```python
from build123d import *

# Parameters (mm, degrees)
BOSS_EXTRUDE1_DEPTH = 100
SKETCH4_W           = 90
SKETCH4_H           = 70
BOSS_EXTRUDE2_DEPTH = 45
SKETCH5_W           = 40
SKETCH5_H           = 45
CUT_EXTRUDE1_DEPTH  = 90
CUT_EXTRUDE2_DEPTH  = 70


with BuildPart() as part:
    # Sketch1 → Boss-Extrude1 (new body)
    with BuildSketch(Plane.XY):
        with BuildLine():
            Line((-52.117117117, 57.815315315), (-52.117117117, 2.815315315))
            Line((-52.117117117, 2.815315315), (47.882882883, 2.815315315))
            Line((47.882882883, 2.815315315), (47.882882883, -22.184684685))
            Line((47.882882883, -22.184684685), (-102.117117117, -22.184684685))
            Line((-102.117117117, -22.184684685), (-102.117117117, 2.815315315))
            Line((-102.117117117, 2.815315315), (-102.117117117, 57.815315315))
            ThreePointArc((-102.117117117, 57.815315315), (-77.117117117, 82.815315315), (-52.117117117, 57.815315315))
        make_face()
        with BuildLine():
            Line((-67.117117117, 57.815315315), (-67.117117117, 2.815315315))
            ThreePointArc((-67.117117117, 2.815315315), (-77.117117117, -7.184684685), (-87.117117117, 2.815315315))
            Line((-87.117117117, 2.815315315), (-87.117117117, 57.815315315))
            ThreePointArc((-87.117117117, 57.815315315), (-77.117117117, 67.815315315), (-67.117117117, 57.815315315))
        make_face(mode=Mode.SUBTRACT)
    extrude(amount=-BOSS_EXTRUDE1_DEPTH)

    # Sketch4 → Boss-Extrude2 (add)
    with BuildSketch(Plane(origin=(0, 2.815315315, 0), x_dir=(1, 0, 0), z_dir=(0, 1, 0))):
        with Locations((-7.117117117, 50)):
            Rectangle(SKETCH4_W, SKETCH4_H)
    extrude(amount=BOSS_EXTRUDE2_DEPTH)

    # Sketch5 → Cut-Extrude1 (cut)
    with BuildSketch(Plane(origin=(37.882882883, 0, 0), x_dir=(0, 0, -1), z_dir=(1, 0, 0))):
        with Locations((50, 25.315315315)):
            Rectangle(SKETCH5_W, SKETCH5_H)
    extrude(amount=-CUT_EXTRUDE1_DEPTH, mode=Mode.SUBTRACT)

    # Sketch6 → Cut-Extrude2 (cut)
    with BuildSketch(Plane.XY.offset(-15)):
        Polygon((-52.117117117, 47.815315315), (37.882882883, 2.815315315), (37.882882883, 47.815315315), align=None)
    extrude(amount=-CUT_EXTRUDE2_DEPTH, mode=Mode.SUBTRACT)


solid = part.part
```
Work out the finished part from the listing and answer in its coordinate system (mm). A direction names the side the tool comes from. Give positions to 0.01 mm unless a question says otherwise; leave off trailing zeros. Write each loop counter-clockwise with the first axis right and the second up, starting at its lowest first coordinate (ties: lowest second). Pieces come first, ordered by that corner, then holes.
(1) The part is cut by section C-C on x = -39. Write down the section's boundary in (y, z).
Final values:
outline: (-22.18, -100) - (2.82, -100) - (2.82, -85) - (41.26, -85) - (41.26, -70) - (2.82, -70) - (2.82, -30) - (41.26, -30) - (41.26, -15) - (2.82, -15) - (2.82, 0) - (-22.18, 0) - close
(2) Which of the six approach directions +Z, -Z, +X, -X, +Y, -Y give full straight-line access (tool end or side, diameter ignored) to faces 4 (the flat face through (-26, 15, -70)), 5 (the flat face through (-18, 20, -15)), 6 (the flat face through (-18, 20, -85)), 7 (the flat face through (-87.117, 30, -49))?
Final values:
face 4: +X, +Y
face 5: +Z, +X, +Y
face 6: -Z, +X, +Y
face 7: +Z, -Z
(3) The part is cut by section B-B on y = -4. Write down the section's boundary in (x, z) (3 decimals).
Final values:
outline: (-102.117, -100) - (-84.435, -100) - (-84.435, 0) - (-102.117, 0) - close; (-69.799, -100) - (47.883, -100) - (47.883, 0) - (-69.799, 0) - close
(4) The part is cut by section A-A on z = -92. Write down the section's boundary in (x, y), plus the area to 3 significant figures.
Final values:
outline: (-102.12, -22.18) - (47.88, -22.18) - (47.88, 2.82) - (-52.12, 2.82) - (-52.12, 57.82) arc R25 ccw to (-102.12, 57.82) - close; hole (-87.12, 2.82) arc R10 ccw to (-67.12, 2.82) - (-67.12, 57.82) arc R10 ccw to (-87.12, 57.82) - close
area: 6,070 mm2
(5) The mould has two halves that part along X. Classify faces 1 (the cylindrical face through (-77.337, 67.813, -49.3)), 2 (the flat face through (-7.75, 25.63, -22.4)), 3 (the flat face through (-26, -22.185, -49)): pulls with the +X half, pulls with the -X half, needs draft (parallel to the pull), parting line crosses it, or undercut.
Final values:
face 1: undercut
face 2: pulls with the +X half
face 3: needs draft
(6) Flat-ended cylindrical pins translate along their axes: pin 1 Ø8 at (x, y) = (-86.5, 66) entering from +Z; pin 2 Ø4 at (x, y) = (30.5, 6.5) entering from -Z; pin 3 Ø12 at (x, z) = (-72, -19) entering from +Y; pin 4 Ø1 at (x, z) = (-36, -68) entering from +Y. Find the tip coordinate at first contact, or state that the pin passes through.
Final values:
pin 1: stops at z = 0
pin 2: stops at z = -85
pin 3: stops at y = 82.82
pin 4: stops at y = 2.82
(7) The part is cut by section D-D on z = -80.5. Write down the section's boundary in (x, y).
Final values:
outline: (-102.12, -22.18) - (47.88, -22.18) - (47.88, 2.82) - (37.88, 2.82) - (-52.12, 47.82) - (-52.12, 57.82) arc R25 ccw to (-102.12, 57.82) - close; hole (-87.12, 2.82) arc R10 ccw to (-67.12, 2.82) - (-67.12, 57.82) arc R10 ccw to (-87.12, 57.82) - close
(8) Straight lines are drawn through the part: line 1 (X direction, y = 23.5, z = -93.5); line 2 (Z direction, x = -22.5, y = 28.5); line 3 (X direction, y = 2, z = -11). For each, find the intervals that lie inside material, in ascending order.
Final values:
line 1: x = -102.12 to -87.12, -67.12 to -52.12
line 2: z = -85 to -70, -30 to -15
line 3: x = -102.12 to -87.08, -67.15 to 47.88
